from build123d import *

# Parameters (mm, degrees)
SKETCH_1_R      = 1.5
SKETCH_1_W      = 10
SKETCH_1_H      = 3
SKETCH_1_W_2    = 9.259227657
SKETCH_1_H_2    = 3.503491546
EXTRUDE_1_DEPTH = 3
FILLET_1_R      = 10


with BuildPart() as part:
    # 草图1 → 凸台-拉伸1 (new body)
    with BuildSketch(Plane(origin=(0, 0, 0), x_dir=(1, 0, 0), z_dir=(0, 1, 0))):
        with BuildLine():
            Line((-49.19123706, -7.5), (49.19123706, -7.5))
            ThreePointArc((49.19123706, -7.5), (65.805615338, 0), (49.19123706, 7.5))
            Line((49.19123706, 7.5), (-49.19123706, 7.5))
            ThreePointArc((-49.19123706, 7.5), (-65.805615338, 0), (-49.19123706, -7.5))
        make_face()
        with Locations(Location((-55.805615338, 0, 0), (0, 0, 270))):
            Circle(SKETCH_1_R, mode=Mode.SUBTRACT)
        with Locations(Location((55.805615338, 0, 0), (0, 0, 270))):
            Circle(SKETCH_1_R, mode=Mode.SUBTRACT)
        with Locations((-15, 0)):
            Rectangle(SKETCH_1_W, SKETCH_1_H, mode=Mode.SUBTRACT)
        with Locations((14.629613829, 0.187687047)):
            Rectangle(SKETCH_1_W_2, SKETCH_1_H_2, mode=Mode.SUBTRACT)
    extrude(amount=EXTRUDE_1_DEPTH)

    # 圆角1
    fillet_1_edges = [part.edges().sort_by_distance(p)[0] for p in [
        (-49.19123706, 1.5, -7.5),
        (49.19123706, 1.5, -7.5),
        (49.19123706, 1.5, 7.5),
        (-49.19123706, 1.5, 7.5),
    ]]
    fillet(fillet_1_edges, radius=FILLET_1_R)


solid = part.part
CAD build for the part. Positions are in the model's coordinates, mm. A direction names the side the tool comes from. Coordinates: 2 decimals unless noted, no trailing zeros. Loops run counter-clockwise (first coordinate to the right, second up) from the corner with the lowest first, then second, coordinate; pieces in that order, holes last. Notation, with made-up numbers: (53, 49) - (71, 49) arc R25 ccw to (71, 64) - close; hole circle Ø11 at (79, 48). An arc over 180 degrees is marked (long way). Use one line per item in the form item = value. Start each with the question number.
1) Band-saw the part on C-C (y = 0.95). Give the cut face in (x, z).
2) Drill centre lines: L1, parallel to X at y = 0.9, z = 0; L2, parallel to Z at x = -19, y = 2.6; L3, parallel to Z at x = 18, y = 1.5. Where is each one in solid material? Low to high. Write a range as from..to.
3) Flat gauge pins, fed straight in: pin 1 (1.5 mm diameter, centred on x = -17, y = 2, fed in from -Z); pin 2 (1.8 mm diameter, centred on x = 55.81, z = 0, fed in from -Y); pin 3 (1.5 mm diameter, centred on x = -13, y = 2, fed in from +Z). Where does each tip first touch, or does it go through?
4) Band-saw the part on B-B (z = 0). Give the cut face in (x, y), and give its area (3 significant figures).
5) Band-saw the part on D-D (x = -13.5). Give the cut face in (y, z), and give its area (3 significant figures).
6) Band-saw the part on A-A (x = 18). Give the cut face in (y, z).
7) Tool access for faces 1 (the face through (-15, 1, -1.5)), 2 (the face through (-1, 3, 0)): list every direction of +Z, -Z, +X, -X, +Y, -Y with a clear straight run to the whole face (end or side of a thin tool).
8) Two-plate mould, pull along Z, no slides. Class faces 3 (the face through (-10, 1, 0)), 4 (the face through (-1, 0, 0)), 5 (the face through (-1, 1, 7.5)), 6 (the face through (1, 1, -7.5)): +Z half, -Z half, draft (parallel to the pull), parting line (faces both ways), or undercut.
Check values:
q1.outline = (-50.96, -8.75) arc R10 cw to (-46.12, -7.5) - (46.12, -7.5) arc R10 cw to (50.96, -8.75) arc R10 ccw (long way) to (50.96, 8.75) arc R10 cw to (46.12, 7.5) - (-46.12, 7.5) arc R10 cw to (-50.96, 8.75) arc R10 ccw (long way) to start; hole circle Ø3 at (-55.81, 0); hole (-20, -1.5) - (-10, -1.5) - (-10, 1.5) - (-20, 1.5) - close; hole (10, -1.94) - (19.26, -1.94) - (19.26, 1.56) - (10, 1.56) - close; hole circle Ø3 at (55.81, 0)
q2.L1 = -65.81..-57.31, -54.31..-20, -10..10, 19.26..54.31, 57.31..65.81
q2.L2 = -7.5..-1.5, 1.5..7.5
q2.L3 = -7.5..-1.94, 1.56..7.5
q3.pin_1 = -7.5
q3.pin_2 = through
q3.pin_3 = 7.5
q4.outline = (-65.81, 0) - (-57.31, 0) - (-57.31, 3) - (-65.81, 3) - close; (-54.31, 0) - (-20, 0) - (-20, 3) - (-54.31, 3) - close; (-10, 0) - (10, 0) - (10, 3) - (-10, 3) - close; (19.26, 0) - (54.31, 0) - (54.31, 3) - (19.26, 3) - close; (57.31, 0) - (65.81, 0) - (65.81, 3) - (57.31, 3) - close
q4.area = 319 mm2
q5.outline = (0, -7.5) - (3, -7.5) - (3, -1.5) - (0, -1.5) - close; (0, 1.5) - (3, 1.5) - (3, 7.5) - (0, 7.5) - close
q5.area = 36.0 mm2
q6.outline = (0, -7.5) - (3, -7.5) - (3, -1.94) - (0, -1.94) - close; (0, 1.56) - (3, 1.56) - (3, 7.5) - (0, 7.5) - close
q7.face_1 = +Y, -Y
q7.face_2 = +Z, -Z, +X, -X, +Y
q8.face_3 = undercut
q8.face_4 = draft
q8.face_5 = +Z half
q8.face_6 = -Z half
